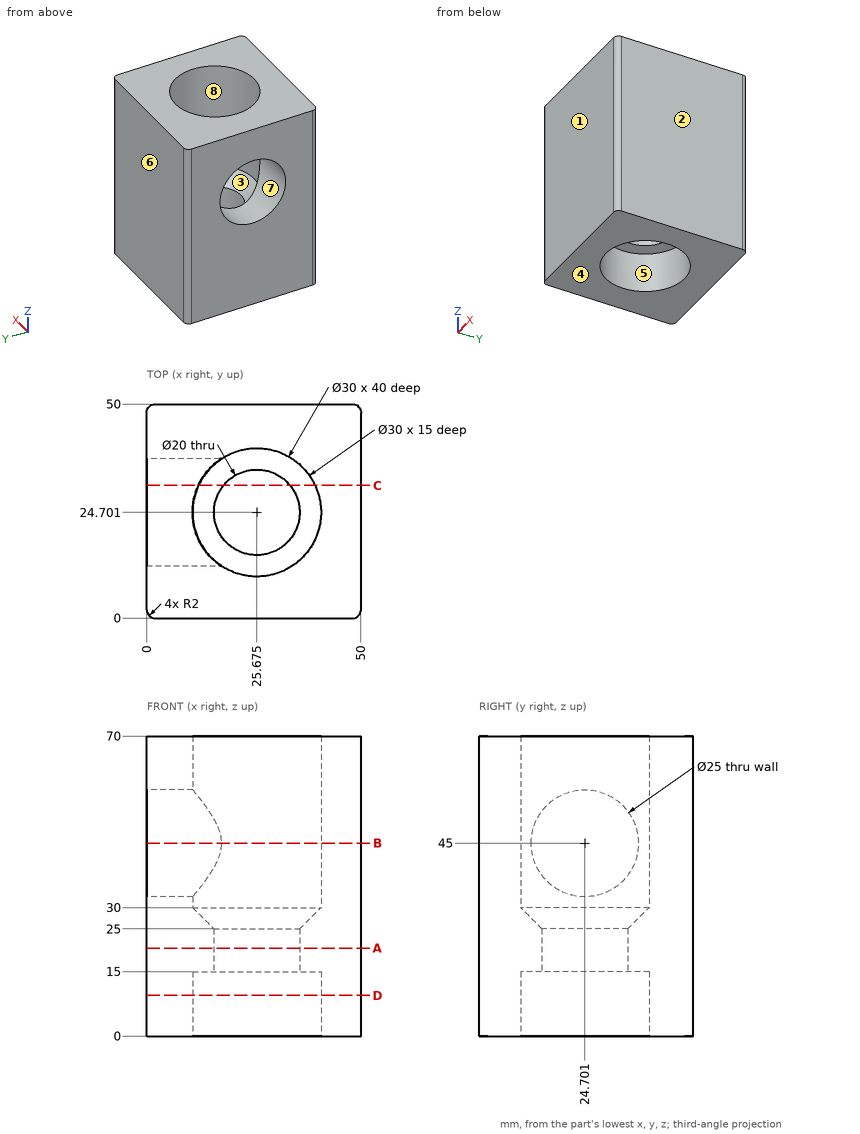
Can you work these out from the drawing? Everything is in mm from the part's minimum corner. A direction names the side the tool comes from. Give positions to 0.01 mm unless a question says otherwise; leave off trailing zeros. Order: outer loops, then holes, each group sorted by start corner. A loop starts at its lowest first (then second) coordinate and runs counter-clockwise, first axis right, second up. Notation, with made-up numbers: M -21,-3.75 L 38,-3.75 A16 cw 38,23.25 Z; hole C -4.5,64 d9. An arc over 180 degrees is marked long. One line per item, written item: value.
Item 1: If we section it at B-B on z = 45: Write out the boundary of the cut face in (x, y) (1 decimal), and give its area (3 significant figures).
Verdict:
outline: M 0,2 A2 ccw 2,0 L 48,0 A2 ccw 50,2 L 50,48 A2 ccw 48,50 L 2,50 A2 ccw 0,48 L 0,37.2 L 17.4,37.2 A15 cw long 17.4,12.2 L 0,12.2 Z
area: 1,470 mm2
Item 2: For pin 1 (3 mm diameter, centred on x = 19, y = 32, fed in from +Z), with a flat end and sliding along its axis, tell me the tip position at first contact or that it passes through.
Verdict:
pin 1: z = 26.39
Item 3: If we section it at C-C on y = 31: State how many separate pieces and enclosed holes the cut face has, and give its area (3 significant figures).
Verdict:
separate pieces: 3
enclosed holes: 0
area: 1,480 mm2
Item 4: For the marked faces 4, 5, 6, 7 and 8, which set-ups out of +Z, -Z, +X, -X, +Y, -Y let a thin tool reach every point of the face, with its end or its side?
Verdict:
face 4: -Z, +X, -X, +Y, -Y
face 5: -Z
face 6: +Z, -Z, +X, -X, +Y
face 7: -X
face 8: +Z
Item 5: If we section it at D-D on z = 9.5: Write out the boundary of the cut face in (x, y) (1 decimal), and give its area (3 significant figures).
Verdict:
outline: M 0,2 A2 ccw 2,0 L 48,0 A2 ccw 50,2 L 50,48 A2 ccw 48,50 L 2,50 A2 ccw 0,48 Z; hole C 25.7,24.7 d30
area: 1,790 mm2
Item 6: If we section it at A-A on z = 20.5: Write out the boundary of the cut face in (x, y) (1 decimal).
Verdict:
outline: M 0,2 A2 ccw 2,0 L 48,0 A2 ccw 50,2 L 50,48 A2 ccw 48,50 L 2,50 A2 ccw 0,48 Z; hole C 25.7,24.7 d20
Item 7: Please list where these lines run through material, in increasing order: line 1 (Y direction, x = 8.75, z = 45); line 2 (X direction, y = 25, z = 39); line 3 (Z direction, x = 3, y = 24.5).
Verdict:
line 1: 0 to 12.2, 37.2 to 50
line 2: 40.67 to 50
line 3: 0 to 32.5, 57.5 to 70
Item 8: If we mould it in two halves opening along X, with no side actions, what happens to the marked faces 1, 2 and 3? For each: pulls with the +X half, pulls with the -X half, needs draft (parallel to the pull), parting line crosses it, or undercut.
Verdict:
face 1: needs draft
face 2: pulls with the +X half
face 3: undercut
